Solid Edge part; units mm, degrees
sketch "Sketch1" plane through (0, 0, 0) normal (0, -1, 0) x (1, 0, 0)
  line L0 (-12, 74) -> (12, 74)
  line L1 (12, 74) -> (12, 24)
  line L2 (12, 24) -> (50, 24)
  line L3 (50, 24) -> (50, 0)
  line L4 (-50, 0) -> (50, 0)
  line L5 (-50, 0) -> (-50, 24)
  line L6 (-50, 24) -> (-12, 24)
  line L7 (-12, 74) -> (-12, 24)
extrude "Protrusion1" add sketch "Sketch1" against normal blind 24
sketch "Sketch2" plane through (50, 12, 12) normal (1, 0, 0) x (0, 1, 0)
  line L0 (-8.35, -8.35) -> (-8.35, 10.5)
  line L1 (-8.35, 10.5) -> (-10.5, 10.5)
  line L2 (-10.5, 10.5) -> (-10.5, -10.5)
  line L3 (-10.5, -10.5) -> (10.5, -10.5)
  line L4 (10.5, -10.5) -> (10.5, -8.35)
  line L5 (10.5, -8.35) -> (-8.35, -8.35)
extrude "Cutout1" cut sketch "Sketch2" against normal through all
sketch "Sketch3" plane through (0, 12, 74) normal (0, 0, 1) x (1, 0, 0)
  line L0 (-8.25, -8.35) -> (8.25, -8.35)
  line L1 (8.25, 8.15) -> (8.25, -8.35)
  line L2 (-8.25, 8.15) -> (8.25, 8.15)
  line L3 (-8.25, -8.35) -> (-8.25, 8.15)
extrude "Cutout2" cut sketch "Sketch3" against normal up to surface (72.5 mm away)
sketch "Sketch4" plane through (-31, 12, 24) normal (0, 0, 1) x (0, -1, 0)
  line L0 (4, 19) -> (4, -19)
  line L1 (4, -19) -> (-4, -19)
  line L2 (-4, 19) -> (-4, -19)
  line L3 (-4, 19) -> (4, 19)
extrude "Protrusion2" add sketch "Sketch4" along normal up to surface (50 mm away)
sketch "Sketch5" plane through (-31, 8, 49) normal (0, -1, 0) x (1, 0, 0)
  line L0 (-11, -25) -> (19, 5)
  line L1 (19, 25) -> (19, 5)
  line L2 (-19, 25) -> (19, 25)
  line L3 (-19, -25) -> (-19, 25)
  line L4 (-11, -25) -> (-19, -25)
extrude "Cutout3" cut sketch "Sketch5" against normal through all
mirror "Mirror1" about plane through (0, 0, 0) normal (1, 0, 0) of "Protrusion2", "Cutout3"
chamfer "Chaflán_1" distance 1.5 angle 45 11 edges at (12, 24, 49) (12, 0, 49) (-12, 0, 49) (-12, 24, 49) (-31, 0, 24) (31, 0, 24) (0, 0, 0) (-31, 24, 24) (31, 24, 24) (0, 24, 0) (29.125, 3.65, 3.65)
sketch "Sketch6" plane through (0, 0, 37.75) normal (0, -1, 0) x (1, 0, 0)
  circle A0 centre (0, 21.25) radius 2.25
  circle A1 centre (0, -25.75) radius 2.25
  circle A2 centre (35, -25.75) radius 2.25
  circle A3 centre (-35, -25.75) radius 2.25
extrude "Cutout5" cut sketch "Sketch6" against normal through all
sketch "Sketch7" plane through (0, 24, 37.75) normal (0, 1, 0) x (-1, 0, 0)
  circle A0 centre (35, -25.75) radius 4
  circle A1 centre (-35, -25.75) radius 4
extrude "VaciadoExtruido_8" cut sketch "Sketch7" against normal blind 8
Verification items for the finished model (mm, model axes). A direction names the side the tool comes from. Give positions to 0.01 mm unless a question says otherwise; leave off trailing zeros. Loops run counter-clockwise (first coordinate to the right, second up) from the corner with the lowest first, then second, coordinate; pieces in that order, holes last.
1) Depth check by flat-ended pin: pin 1 Ø10 at (x, z) = (35.5, 18) entering from -Y; pin 2 Ø2 at (y, z) = (9, 52.5) entering from -X; pin 3 Ø2 at (y, z) = (4, 56.5) entering from +X; pin 4 Ø3.5 at (x, z) = (35, 12) entering from -Y. Enter the tip coordinate at first touch or a pass-through.
2) Set-up check for faces 1 (the flat face through (21, 16, 32)), 2 (the flat face through (1, 22.5, 3)), 3 (the flat face through (-31, 7, 24)): record each of +Z, -Z, +X, -X, +Y, -Y from which the full face is reachable in a straight line by a thin tool's end or side.
3) Sectioned sample at A-A, the plane y = 11. Enter the section's corners in (x, z), then the cut area to 3 significant figures.
4) Draft check along Y on faces 4 (the flat face through (0, 3.65, 49)), 5 (the cylindrical face through (36.21, 9.739, 13.897)), 6 (the flat face through (33, 16, 14)). Enter one of: pulls with the +Y half, pulls with the -Y half, needs draft (parallel to the pull), parting line crosses it, or undercut.
5) Sectioned sample at B-B, the plane x = 0. Count the separate pieces of the cut face and the enclosed holes in it, then the cut area to 3 significant figures.
6) Thickness scan on line 1 along Z through (x, y) = (0, 21.25); line 2 along Z through (x, y) = (-35, 21.25); line 3 along Y through (x, z) = (-35, 7.5). Record the ranges inside material, lowest first.
7) Sectioned sample at D-D, the plane x = -22. Enter the section's corners in (y, z), then the cut area to 3 significant figures.
8) Sectioned sample at C-C, the plane z = 46.5. Enter the section's corners in (x, y), then the cut area to 3 significant figures.
Answers:
1. pin 1: stops at y = 0
1. pin 2: stops at x = -14.5
1. pin 3: stops at x = 12
1. pin 4: passes through
2. face 1: +Z, +X, +Y
2. face 2: +X, -X
2. face 3: +Z, -X
3. outline: (-50, 0) - (50, 0) - (50, 1.5) - (-50, 1.5) - close; (-50, 3.65) - (-8.25, 3.65) - (-8.25, 74) - (-12, 74) - (-12, 54) - (-42, 24) - (-50, 24) - close; (8.25, 3.65) - (50, 3.65) - (50, 24) - (42, 24) - (12, 54) - (12, 74) - (8.25, 74) - close; hole circle Ø4.5 at (-35, 12); hole circle Ø4.5 at (35, 12)
3. area: 3,090 mm2
4. face 4: undercut
4. face 5: needs draft
4. face 6: pulls with the +Y half
5. separate pieces: 5
5. enclosed holes: 0
5. area: 469 mm2
6. line 1: z = 0 to 1.5, 3.65 to 9.75, 14.25 to 56.75, 61.25 to 74
6. line 2: z = 0 to 1.5, 3.65 to 8, 16 to 24
6. line 3: y = 0 to 1.5, 3.65 to 24
7. outline: (0, 1.5) - (1.5, 0) - (22.5, 0) - (24, 1.5) - (24, 22.5) - (22.5, 24) - (16, 24) - (16, 44) - (8, 44) - (8, 24) - (1.5, 24) - (0, 22.5) - close; hole (1.5, 1.5) - (22.5, 1.5) - (22.5, 3.65) - (3.65, 3.65) - (3.65, 22.5) - (1.5, 22.5) - close
7. area: 646 mm2
8. outline: (-19.5, 8) - (-12, 8) - (-12, 1.5) - (-10.5, 0) - (10.5, 0) - (12, 1.5) - (12, 8) - (19.5, 8) - (19.5, 16) - (12, 16) - (12, 22.5) - (10.5, 24) - (-10.5, 24) - (-12, 22.5) - (-12, 16) - (-19.5, 16) - close; hole (-8.25, 3.65) - (8.25, 3.65) - (8.25, 20.15) - (-8.25, 20.15) - close
8. area: 419 mm2
